CAD build for the part. Positions are in the model's coordinates, mm. Face numbers are marked on the shaded views. Give positions to 0.01 mm unless a question says otherwise; leave off trailing zeros. Loops run counter-clockwise (first coordinate to the right, second up) from the corner with the lowest first, then second, coordinate; pieces in that order, holes last. Notation, with made-up numbers: M -31,-12 L 19,-12 A23 ccw 19,5 Z; hole C -31.75,44 d8. An arc over 180 degrees is marked long. Answer as CSV lines item,"result".
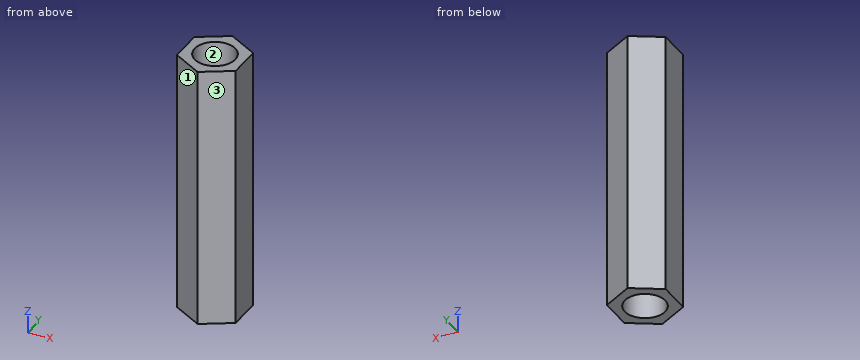
Autodesk Inventor part; units mm, degrees
ref_plane "YZ Plane" through (0, 0, 0) normal (1, 0, 0) x (0, 1, 0)
ref_plane "XZ Plane" through (0, 0, 0) normal (0, 1, 0) x (-1, 0, 0)
ref_plane "XY Plane" through (0, 0, 0) normal (0, 0, 1) x (1, 0, 0)
sketch "Эскиз1" plane through (0, 0, 0) normal (0, 0, 1) x (1, 0, 0)
  line L0 (0, 2.5) -> (2.1651, 1.25)
  line L1 (2.1651, 1.25) -> (2.1651, -1.25)
  line L2 (2.1651, -1.25) -> (0, -2.5)
  line L3 (0, -2.5) -> (-2.1651, -1.25)
  line L4 (-2.1651, -1.25) -> (-2.1651, 1.25)
  line L5 (-2.1651, 1.25) -> (0, 2.5)
  point P0 (0, 0)
  point P1 (0, 0)
  dimension "d0" = 5
extrude "Выдавливание1" add sketch "Эскиз1" against normal blind 19.5
sketch "Эскиз2" plane through (0, 0, 0) normal (0, 0, 1) x (1, 0, 0)
  circle A0 centre (0, 0) radius 1.5
  dimension "d3" = 3
extrude "Выдавливание2" cut sketch "Эскиз2" against normal through all
thread "Резьба1"
properties part number "Кусок металла"
1) Band-saw the part on B-B on z = -7. Give the cut face in (x, y).
Answer below:
outline,"M -2.17,-1.25 L 0,-2.5 L 2.17,-1.25 L 2.17,1.25 L 0,2.5 L -2.17,1.25 Z; hole C 0,0 d3"
2) Mould opens along X. For the marked faces 1, 2 and 3 say: +X half, -X half, draft (parallel to the pull), parting line (faces both ways), or undercut.
Answer below:
face 1,"-X half"
face 2,"undercut"
face 3,"+X half"
3) Band-saw the part on D-D on x = 1.7. Give the cut face in (y, z), and give its area (3 significant figures).
Answer below:
outline,"M -1.52,-19.5 L 1.52,-19.5 L 1.52,0 L -1.52,0 Z"
area,"59.2 mm^2"
4) Band-saw the part on A-A on y = 0. Give the cut face in (x, z), and give its area (3 significant figures).
Answer below:
outline,"M -2.17,-19.5 L -1.5,-19.5 L -1.5,0 L -2.17,0 Z; M 1.5,-19.5 L 2.17,-19.5 L 2.17,0 L 1.5,0 Z"
area,"25.9 mm^2"
5) Flat gauge pins, fed straight in: pin 1 (1 mm diameter, centred on x = -1.5, z = -15, fed in from -Y); pin 2 (1.5 mm diameter, centred on x = -1, z = -6.5, fed in from -Y). Where does each tip first touch, or does it go through?
Answer below:
pin 1,"stops at y = -1.92"
pin 2,"stops at y = -2.36"
6) Drill centre lines: line 1 (X direction, y = 0.1, z = -13.75); line 2 (Y direction, x = 0.85, z = -6); line 3 (Y direction, x = -0.75, z = -1.5). Where is each one in solid material? Low to high. Write a range as from..to.
Answer below:
line 1,"x = -2.17..-1.5, 1.5..2.17"
line 2,"y = -2.01..-1.24, 1.24..2.01"
line 3,"y = -2.07..-1.3, 1.3..2.07"
7) Band-saw the part on C-C on x = 0.2. Give the cut face in (y, z), and give its area (3 significant figures).
Answer below:
outline,"M -2.38,-19.5 L -1.49,-19.5 L -1.49,0 L -2.38,0 Z; M 1.49,-19.5 L 2.38,-19.5 L 2.38,0 L 1.49,0 Z"
area,"35.0 mm^2"
